Here's how the part is built. I have some questions about the finished solid (model axes, mm). Face numbers are marked on the shaded views. Give positions to 0.01 mm unless a question says otherwise; leave off trailing zeros. Loops run counter-clockwise (first coordinate to the right, second up) from the corner with the lowest first, then second, coordinate; pieces in that order, holes last. Notation, with made-up numbers: (-39.75, 42) - (-10.75, 42) arc R16 cw to (-10.75, 60) - close; hole circle Ø6 at (-18.75, 40.25). An arc over 180 degrees is marked (long way). Use a Markdown table: item, result.
from build123d import *

# Parameters (mm, degrees)
SKETCH1_R           = 3
BOSS_EXTRUDE1_DEPTH = 20
FILLET1_R           = 0.2


with BuildPart() as part:
    # Sketch1 → Boss-Extrude1 (new body)
    with BuildSketch(Plane(origin=(0, 0, 0), x_dir=(1, 0, 0), z_dir=(0, 1, 0))):
        with Locations(Location((0, 0, 0), (0, 0, 270))):
            Circle(SKETCH1_R)
    extrude(amount=BOSS_EXTRUDE1_DEPTH)

    # Fillet1
    fillet1_edges = [part.edges().sort_by_distance(p)[0] for p in [
        (0, 0, -3),
        (0, 20, -3),
    ]]
    fillet(fillet1_edges, radius=FILLET1_R)

    # Sketch3 → M3x0.5 Tapped Hole1 (revolve, cut)
    with BuildSketch(Plane(origin=(0, 20, 0), x_dir=(0, 0, 1), z_dir=(1, 0, 0))):
        Polygon((0, 0), (0, 20), (1.525, 20), (1.25, 19.725), (1.25, 0.275), (1.525, 0), align=None)
    revolve(axis=Axis((0, 26.35, 0), (0, -1, 0)), mode=Mode.SUBTRACT)


solid = part.part
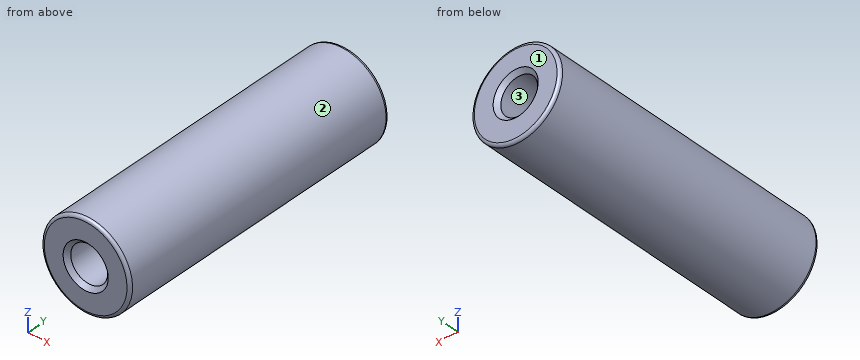
(1) Suppose I cut it at C-C on y = 4.75. Write out the boundary of the cut face in (x, z).
A:
| item | result |
|---|---|
| outline | circle Ø6 at (0, 0); hole circle Ø2.5 at (0, 0) |
(2) Suppose I cut it at B-B on z = 0. Write out the boundary of the cut face in (x, y) (3 decimals).
A:
| item | result |
|---|---|
| outline | (-3, 0.2) arc R0.2 ccw to (-2.8, 0) - (-1.525, 0) - (-1.25, 0.275) - (-1.25, 19.725) - (-1.525, 20) - (-2.8, 20) arc R0.2 ccw to (-3, 19.8) - close; (1.25, 0.275) - (1.525, 0) - (2.8, 0) arc R0.2 ccw to (3, 0.2) - (3, 19.8) arc R0.2 ccw to (2.8, 20) - (1.525, 20) - (1.25, 19.725) - close |
(3) Suppose I cut it at A-A on x = 0. Write out the boundary of the cut face in (y, z) (3 decimals), plus the area to 3 significant figures.
A:
| item | result |
|---|---|
| outline | (0, -2.8) arc R0.2 ccw to (0.2, -3) - (19.8, -3) arc R0.2 ccw to (20, -2.8) - (20, -1.525) - (19.725, -1.25) - (0.275, -1.25) - (0, -1.525) - close; (0, 1.525) - (0.275, 1.25) - (19.725, 1.25) - (20, 1.525) - (20, 2.8) arc R0.2 ccw to (19.8, 3) - (0.2, 3) arc R0.2 ccw to (0, 2.8) - close |
| area | 69.8 mm2 |
(4) We'd pull the mould along Z, two halves only. Please class the marked faces 1, 2 and 3: pulls with the +Z half, pulls with the -Z half, needs draft (parallel to the pull), parting line crosses it, or undercut.
A:
| item | result |
|---|---|
| face 1 | needs draft |
| face 2 | parting line crosses it |
| face 3 | undercut |
(5) Will these pins go through, and if not, where does the flat tip stop? pin 1 (3 mm diameter, centred on x = 0, z = 0, fed in from -Y) (3 decimals); pin 2 (1.5 mm diameter, centred on y = 16, z = -2, fed in from -X); pin 3 (2 mm diameter, centred on y = 2.5, z = 0.5, fed in from -X).
A:
| item | result |
|---|---|
| pin 1 | y = 0.025 |
| pin 2 | x = -2.73 |
| pin 3 | x = -3 |
(6) If I drill on line 1 (X direction, y = 6.25, z = 0); line 2 (Z direction, x = 0.5, y = 6.75); line 3 (X direction, y = 14.5, z = 1), over which ranges is the centre line in solid material (lowest first)?
A:
| item | result |
|---|---|
| line 1 | -3 to -1.25, 1.25 to 3 |
| line 2 | -2.96 to -1.15, 1.15 to 2.96 |
| line 3 | -2.83 to -0.75, 0.75 to 2.83 |
